from build123d import *

# Parameters (mm, degrees)
F2_R     = 12.7
F3_DEPTH = 127
F4_R     = 6.35
F5_DEPTH = 127
F7_DEPTH = 127
F7_TAPER = 1
F9_DEPTH = 63.5


with BuildPart() as f1:
    # F0 (on Front) → F1 (revolve)
    with BuildSketch(Plane.XZ):
        with BuildLine():
            ThreePointArc((0, -63.5), (44.9012806053, -44.9012806053), (63.5, 0))
            ThreePointArc((63.5, 0), (44.9012806053, 44.9012806053), (0, 63.5))
            Line((0, 63.5), (0, -63.5))
        make_face()
    revolve(axis=Axis((0, 0, 0), (0, 0, -1)))

    # F2 (on Front) → F3 (join)
    with BuildSketch(Plane.XZ):
        Circle(F2_R)
    extrude(amount=F3_DEPTH)

    # F4 (on Front) → F5 (cut, symmetric)
    with BuildSketch(Plane.XZ):
        Circle(F4_R)
    extrude(amount=F5_DEPTH, both=True, mode=Mode.SUBTRACT)

    # F6 (on Front) → F7 (join)
    with BuildSketch(Plane.XZ):
        Polygon((-17.4312744727, -10.324512409), (-8.0336011509, -18.5985520613), (4.4326347585, -19.7685769676), (2.7486874728, -12.2585421145), (0.2662621749, -13.1211935126), (-7.4970334147, -10.7717735178), (-12.3967170547, -4.3079021583), (-12.5612761287, 3.8014414054), (-7.9278546636, 10.4587635585), (-2.7486874728, 12.2585421145), (-4.4326347585, 19.7685769676), (-15.2057548499, 13.3876773816), (-20.1707934132, 1.8931400662), align=None)
        Polygon((2.7486874728, -12.2585421145), (4.4326347585, -19.7685769676), (15.2057548499, -13.3876773816), (20.1707934132, -1.8931400662), (17.4312744727, 10.324512409), (8.0336011509, 18.5985520613), (-4.4326347585, 19.7685769676), (-2.7486874728, 12.2585421145), (-0.2662621749, 13.1211935126), (7.4970334147, 10.7717735178), (12.3967170547, 4.3079021583), (12.5612761287, -3.8014414054), (7.9278546636, -10.4587635585), align=None)
    extrude(amount=-F7_DEPTH, taper=F7_TAPER)

    # F8 (on Top) → F9 (cut, symmetric)
    with BuildSketch(Plane.XY):
        Polygon((-6.0909675368, -8.3834975958), (6.0909675368, -8.3834975958), (9.8553924989, 3.202211137), (0, 10.3625729176), (-9.8553924989, 3.202211137), align=None)
    extrude(amount=F9_DEPTH, both=True, mode=Mode.SUBTRACT)


solid = f1.part
Here's how the part is built. I have some questions about the finished solid (model axes, mm). A direction names the side the tool comes from. Give positions to 0.01 mm unless a question says otherwise; leave off trailing zeros. Order: outer loops, then holes, each group sorted by start corner. A loop starts at its lowest first (then second) coordinate and runs counter-clockwise, first axis right, second up. Notation, with made-up numbers: (57.5, 1) -> (64.5, 1) arc R11 cw to (64.5, 11) -> close; hole circle Ø9 at (67.5, 61). An arc over 180 degrees is marked (long way). One line per item, written item: value. Start each with the question number.
1. We'd pull the mould along Y, two halves only. Please class faces 1 (the face through (12, 127, -9)), 2 (the face through (-7.05, 5.24, 0.88)), 3 (the face through (3.414, -68.049, 5.354)), 4 (the face through (7.947, -2.672, 0.881)): released by +Y, released by -Y, zero draft, split by the parting line, or undercut.
2. Imagine slicing it at B-B, the plane z = -51. List the corners of the cut face in (x, y) for me.
3. Will these pins go through, and if not, where does the flat tip stop? pin 1 Ø10 at (y, z) = (-31, 18) entering from -X; pin 2 Ø8 at (x, y) = (15.5, 41.5) entering from +Z; pin 3 Ø5 at (y, z) = (-90.5, 6.5) entering from -X; pin 4 Ø11.5 at (x, z) = (0, 0) entering from -Y.
4. Imagine slicing it at D-D, the plane x = 40.5. List the corners of the cut face in (y, z) for me, plus the area to 3 significant figures.
5. Imagine slicing it at C-C, the plane z = 40. List the corners of the cut face in (x, y) for me.
6. I need wall thicknesses on probe 1 along Z at (x, y) = (0, -101); probe 2 along X at (y, z) = (-35, 0); probe 3 along Z at (x, y) = (0, 41). Which ranges of each line are inside material? Lowest first, please. Write a range as from..to.
7. Imagine slicing it at A-A, the plane y = -101. List the corners of the cut face in (x, z) for me, plus the area to 3 significant figures.
8. For faces 5 (the face through (-2.75, -94.16, -12.4)), 6 (the face through (6.057, 34.063, 1.907)), 7 (the face through (0, -8.383, -32)), which set-ups out of +Z, -Z, +X, -X, +Y, -Y let a thin tool reach every point of the face, with its end or its side?
Values follow:
1. face 1: released by +Y
1. face 2: undercut
1. face 3: zero draft
1. face 4: undercut
2. outline: circle Ø75.66 at (0, 0); hole (-9.86, 3.2) -> (-6.09, -8.38) -> (6.09, -8.38) -> (9.86, 3.2) -> (0, 10.36) -> close
3. pin 1: stops at x = -55.5
3. pin 2: stops at z = 49.07
3. pin 3: stops at x = -12.05
3. pin 4: passes through
4. outline: circle Ø97.82 at (0, 0)
4. area: 7,510 mm2
5. outline: circle Ø98.64 at (0, 0); hole (-9.86, 3.2) -> (-6.09, -8.38) -> (6.09, -8.38) -> (9.86, 3.2) -> (0, 10.36) -> close
6. probe 1: z = -12.7..-6.35, 6.35..12.7
6. probe 2: x = -52.98..-6.35, 6.35..52.98
6. probe 3: z = -48.49..-6.35, 6.35..48.49
7. outline: circle Ø25.4 at (0, 0); hole circle Ø12.7 at (0, 0)
7. area: 380 mm2
8. face 5: -Y
8. face 6: +Y, -Y
8. face 7: +Z, -Z
